CAD build for the part. Positions are in the model's coordinates, mm. Face numbers are marked on the shaded views. A direction names the side the tool comes from. Give positions to 0.01 mm unless a question says otherwise; leave off trailing zeros. Loops run counter-clockwise (first coordinate to the right, second up) from the corner with the lowest first, then second, coordinate; pieces in that order, holes last.
```python
from build123d import *

# Parameters (mm, degrees)
SKETCH1_W           = 95.25
SKETCH1_H           = 38.1
BOSS_EXTRUDE1_DEPTH = 3.175
SKETCH2_W           = 38.1
SKETCH2_H           = 38.1
BOSS_EXTRUDE2_DEPTH = 3.175
SKETCH3_R           = 7.3025
CUT_EXTRUDE2_DEPTH  = 39.1
SKETCH4_R           = 8.001
CUT_EXTRUDE3_DEPTH  = 4.175
FILLET1_R           = 2.54


with BuildPart() as part:
    # Sketch1 → Boss-Extrude1 (new body)
    with BuildSketch(Plane(origin=(0, 0, 0), x_dir=(1, 0, 0), z_dir=(0, 1, 0))):
        Rectangle(SKETCH1_W, SKETCH1_H)
    extrude(amount=BOSS_EXTRUDE1_DEPTH)

    # Sketch2 → Boss-Extrude2 (add)
    with BuildSketch(Plane.ZY.offset(47.625)):
        with Locations((0, 19.05)):
            Rectangle(SKETCH2_W, SKETCH2_H)
    extrude(amount=BOSS_EXTRUDE2_DEPTH)

    # Sketch3 → Cut-Extrude2 (cut, through all)
    with BuildSketch(Plane(origin=(0, 0, 0), x_dir=(1, 0, 0), z_dir=(0, 1, 0))):
        with Locations((26.035, 0)):
            Circle(SKETCH3_R)
    extrude(amount=CUT_EXTRUDE2_DEPTH, mode=Mode.SUBTRACT)

    # Sketch4 → Cut-Extrude3 (cut, through all)
    with BuildSketch(Plane.ZY.offset(47.625)):
        with Locations((0, 15.875)):
            Circle(SKETCH4_R)
    extrude(amount=CUT_EXTRUDE3_DEPTH, mode=Mode.SUBTRACT)

    # Fillet1
    fillet1_edges = [part.edges().sort_by_distance(p)[0] for p in [
        (-47.625, 3.175, 0),
        (-50.8, 0, 0),
    ]]
    fillet(fillet1_edges, radius=FILLET1_R)


solid = part.part
```
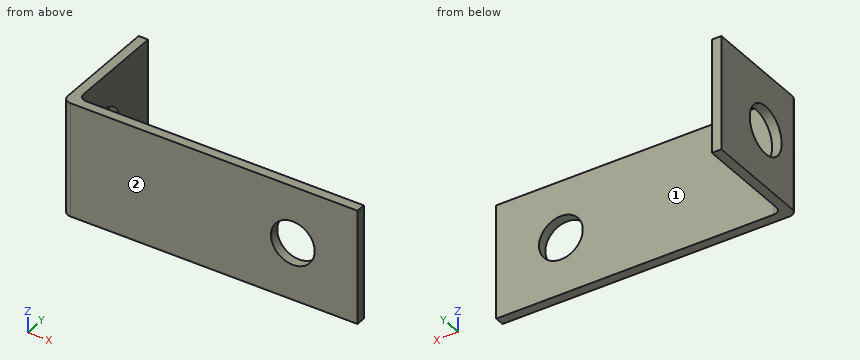
1. Saw through at B-B, the plane y = 12. List the corners of the cut face in (x, z) (3 decimals).
Responses:
outline: (-50.8, -19.05) - (-47.625, -19.05) - (-47.625, -7) - (-50.8, -7) - close; (-50.8, 7) - (-47.625, 7) - (-47.625, 19.05) - (-50.8, 19.05) - close
2. Saw through at D-D, the plane z = 0. List the corners of the cut face in (x, y) (1 decimal), and give its area (3 significant figures).
Responses:
outline: (-50.8, 2.5) arc R2.5 ccw to (-48.3, 0) - (18.7, 0) - (18.7, 3.2) - (-45.1, 3.2) arc R2.5 cw to (-47.6, 5.7) - (-47.6, 7.9) - (-50.8, 7.9) - close; (-50.8, 23.9) - (-47.6, 23.9) - (-47.6, 38.1) - (-50.8, 38.1) - close; (33.3, 0) - (47.6, 0) - (47.6, 3.2) - (33.3, 3.2) - close
area: 326 mm2
3. Drop flat-ended pins along their axis: pin 1 (10 mm diameter, centred on y = 19, z = 13.5, fed in from +X) (3 decimals); pin 2 (8 mm diameter, centred on x = 32, z = -7, fed in from +Y) (3 decimals). Give the stop position or say it passes through.
Responses:
pin 1: stops at x = -47.625
pin 2: stops at y = 3.175
4. Probe line 1 along Y through (x, z) = (-48, 0); line 2 along Y through (x, z) = (40.5, -10) (3 decimals); line 3 along X through (y, z) = (27.5, -5.5) (3 decimals). List the from-to ranges inside material, lowest first.
Responses:
line 1: y = 0 to 7.87, 23.88 to 38.1
line 2: y = 0 to 3.175
line 3: x = -50.8 to -47.625
5. Saw through at A-A, the plane z = 13. List the corners of the cut face in (x, y) (3 decimals).
Responses:
outline: (-50.8, 2.54) arc R2.54 ccw to (-48.26, 0) - (47.625, 0) - (47.625, 3.175) - (-45.085, 3.175) arc R2.54 cw to (-47.625, 5.715) - (-47.625, 38.1) - (-50.8, 38.1) - close
6. Tool access for the marked faces 1 and 2: list every direction of +Z, -Z, +X, -X, +Y, -Y with a clear straight run to the whole face (end or side of a thin tool).
Responses:
face 1: +Z, -Z, +X, +Y
face 2: +Z, -Z, +X, -X, -Y
7. Saw through at C-C, the plane x = 25.5. List the corners of the cut face in (y, z) (3 decimals), and give its area (3 significant figures).
Responses:
outline: (0, -19.05) - (3.175, -19.05) - (3.175, -7.283) - (0, -7.283) - close; (0, 7.283) - (3.175, 7.283) - (3.175, 19.05) - (0, 19.05) - close
area: 74.7 mm2
